Autodesk Inventor part; units mm, degrees
ref_plane "YZ Plane" through (0, 0, 0) normal (1, 0, 0) x (0, 1, 0)
ref_plane "XZ Plane" through (0, 0, 0) normal (0, 1, 0) x (-1, 0, 0)
ref_plane "XY Plane" through (0, 0, 0) normal (0, 0, 1) x (1, 0, 0)
sketch "Sketch1" plane through (0, 0, 0) normal (1, 0, 0) x (0, 1, 0)
  line L0 (10.2056, -9.9502) -> (10.2056, -91.7507)
  arc A0 (10.2056, -9.9502) -> (3.8556, -9.9502) centre (7.0306, -6.4004) ccw
  arc A1 (3.8556, -91.7507) -> (10.2056, -91.7507) centre (7.0306, -95.3004) ccw
  line L1 (3.8556, -9.9502) -> (3.8556, -91.7507)
  point P0 (0, 0)
  dimension "d1" = 88.9
  dimension "d2" = 9.525
  dimension "d5" = 6.35
  dimension "d6" = 9.525
  dimension "d7" = 0
  dimension "d8" = 3.175
extrude "Extrusion1" add sketch "Sketch1" along normal blind 3.175
sketch "Sketch2" plane through (3.175, 0, 0) normal (1, 0, 0) x (0, 0, -1)
  arc A0 (9.9502, 10.2056) -> (9.9502, 3.8556) centre (6.4004, 7.0306) ccw
  arc A1 (91.7507, 3.8556) -> (91.7507, 10.2056) centre (95.3004, 7.0306) ccw
  point P0 (0, 0)
hole "Hole1" at (3.175, 7.0306, -6.4004) at (3.175, 7.0306, -95.3004) direction (-1, 0, 0) diameter 3.2512 depth 25.4 tip angle 118
properties part number "Linkage Arm"
Work out the finished part from the listing and answer in its coordinate system (mm). Round coordinates to 2 decimals unless told otherwise and drop trailing zeros. Order: outer loops, then holes, each group sorted by start corner. A loop starts at its lowest first (then second) coordinate and runs counter-clockwise, first axis right, second up. Notation, with made-up numbers: M 60.5,22.5 L 105.5,22.5 A23 cw 105.5,55.5 Z; hole C 36.5,24.5 d5. An arc over 180 degrees is marked long. One line per item, written item: value.
Q1. Flat-ended cylindrical pins translate along their axes: pin 1 (1 mm diameter, centred on x = 1.5, y = 9.5, fed in from -Z); pin 2 (1 mm diameter, centred on y = 9, z = -27, fed in from -X); pin 3 (1.6 mm diameter, centred on x = 1, z = -51, fed in from -Y); pin 4 (1 mm diameter, centred on x = 1, z = -68, fed in from +Y). Find the tip coordinate at first contact, or state that the pin passes through.
Derived:
pin 1: z = -99.64
pin 2: x = 0
pin 3: y = 3.86
pin 4: y = 10.21
Q2. Find section B-B on z = -11. Write down the section's boundary in (x, y) (3 decimals), then the cut area to 3 significant figures.
Derived:
outline: M 0,3.856 L 3.175,3.856 L 3.175,10.206 L 0,10.206 Z
area: 20.2 mm²
Q3. Straight lines are drawn through the part: line 1 (Z direction, x = 2.85, y = 7.25); line 2 (Z direction, x = 2.2, y = 7.75); line 3 (Y direction, x = 1.4, z = -26). For each, find the intervals that lie inside material, in ascending order.
Derived:
line 1: -100.06 to -96.91, -93.69 to -8.01, -4.79 to -1.64
line 2: -100.01 to -96.76, -93.84 to -7.86, -4.94 to -1.69
line 3: 3.86 to 10.21
Q4. Find section A-A on x = 2.55. Write down the section's boundary in (y, z).
Derived:
outline: M 3.86,-91.75 A4.76 ccw long 10.21,-91.75 L 10.21,-9.95 A4.76 ccw long 3.86,-9.95 Z; hole C 7.03,-95.3 d3.25; hole C 7.03,-6.4 d3.25
Q5. Determine the mould class of faces 1 (the face through (2, 10.206, -50)), 2 (the face through (3.175, 7, -50)), 3 (the face through (1.565, 7.653, -96.802)), 4 (the face through (2, 3.856, -50)) for opening direction Y: released by +Y, released by -Y, zero draft, split by the parting line, or undercut.
Derived:
face 1: released by +Y
face 2: zero draft
face 3: undercut
face 4: released by -Y
